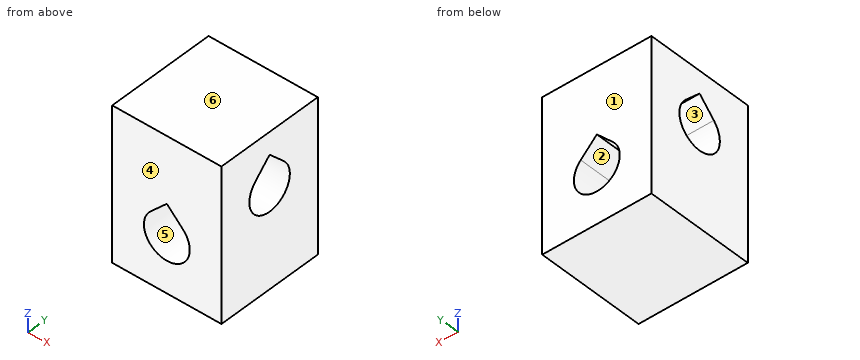
Solid Edge part; units mm, degrees
sketch "Sketch1" plane through (0, 0, 0) normal (0, 0, 1) x (1, 0, 0)
  line L0 (-10, -10) -> (10, -10)
  line L1 (10, -10) -> (10, 10)
  line L2 (10, 10) -> (-10, 10)
  line L3 (-10, 10) -> (-10, -10)
  dimension "D1" = 10
  dimension "D2" = 10
extrude "Protrusion1" add sketch "Sketch1" along normal mid plane 28
sketch "Sketch2" plane through (0, -10, 12) normal (0, -1, 0) x (1, 0, 0)
  circle A0 centre (0, -16) radius 4.2
extrude "Cutout1" cut sketch "Sketch2" against normal through all
sketch "Sketch3" plane through (10, 0, 0) normal (1, 0, 0) x (0, 1, 0)
  circle A0 centre (0, 4) radius 4.2
extrude "Cutout2" cut sketch "Sketch3" against normal through all
sketch "Sketch4" plane through (0, -10, 0) normal (0, -1, 0) x (1, 0, 0)
  line L0 (0, -4) -> (2.9698, -1.0302)
  line L1 (2.9698, -1.0302) -> (0, 1.9397)
  line L2 (0, 1.9397) -> (-2.9698, -1.0302)
  line L3 (-2.9698, -1.0302) -> (0, -4)
extrude "Cutout3" cut sketch "Sketch4" against normal through all
sketch "Sketch5" plane through (10, 0, 0) normal (1, 0, 0) x (0, 1, 0)
  line L0 (0, 4) -> (2.9698, 6.9698)
  line L1 (2.9698, 6.9698) -> (0, 9.9397)
  line L2 (0, 9.9397) -> (-2.9698, 6.9698)
  line L3 (-2.9698, 6.9698) -> (0, 4)
extrude "Cutout4" cut sketch "Sketch5" against normal through all
extrude "Cutout5" [suppressed]
extrude "Cutout6" [suppressed]
Input: part model. Units: mm. Frame: model coordinates. Face numbers are marked on the shaded views. A direction names the side the tool comes from. Give positions to 0.01 mm unless a question says otherwise; leave off trailing zeros. Order: outer loops, then holes, each group sorted by start corner. A loop starts at its lowest first (then second) coordinate and runs counter-clockwise, first axis right, second up.
1. Section B-B on z = -4. Return the cut outline in (x, y).
Derived:
outline: (-10, -10) - (-4.2, -10) - (-4.2, 10) - (-10, 10) - close; (4.2, -10) - (10, -10) - (10, 10) - (4.2, 10) - close
2. Material intervals for L1, parallel to Z at x = -2.25, y = -1.75; L2, parallel to X at y = -3.25, z = -4; L3, parallel to X at y = 8, z = -3, sorted ascending.
Derived:
L1: z = -14 to -7.55, -0.31 to 0.18, 8.19 to 14
L2: x = -10 to -4.2, 4.2 to 10
L3: x = -10 to -4.08, 4.08 to 10
3. Section C-C on z = 3.25. Return the cut outline in (x, y).
Derived:
outline: (-10, -10) - (10, -10) - (10, -4.13) - (-10, -4.13) - close; (-10, 4.13) - (10, 4.13) - (10, 10) - (-10, 10) - close
4. Section A-A on x = 5.5. Return the cut outline in (y, z), and give its area (3 significant figures).
Derived:
outline: (-10, -14) - (10, -14) - (10, 14) - (-10, 14) - close; hole (-2.95, 6.99) arc R4.2 ccw (long way) to (2.95, 6.99) - (0, 9.94) - close
area: 501 mm2
5. Mould query, pull axis Z, two halves, no side actions, for the marked faces 4, 5 and 6. Classes: released by +Z, released by -Z, zero draft, split by the parting line, or undercut.
Derived:
face 4: zero draft
face 5: undercut
face 6: released by +Z
6. Reachability of the marked faces 1, 2 and 3 from +Z, -Z, +X, -X, +Y, -Y: full face, straight path, thin tool, end or side. Return the list, or none.
Derived:
face 1: +Z, -Z, +X, -X, +Y
face 2: +Y, -Y
face 3: +X, -X
